```python
from build123d import *

# Parameters (mm, degrees)
EXTRUDE_1_DEPTH = 0.5
EXTRUDE_2_DEPTH = 0.2


with BuildPart() as part:
    # Эскиз1 → Бобышка-Вытянуть1 (new body)
    with BuildSketch(Plane.XY):
        with BuildLine():
            Line((25.396850198, 14), (-25.396850198, 14))
            ThreePointArc((-25.396850198, 14), (-29, 0), (-25.396850198, -14))
            Line((-25.396850198, -14), (25.396850198, -14))
            ThreePointArc((25.396850198, -14), (29, 0), (25.396850198, 14))
        make_face()
    extrude(amount=EXTRUDE_1_DEPTH)

    # Эскиз2 → Бобышка-Вытянуть2 (add)
    with BuildSketch(Plane(origin=(0, 0, 0), x_dir=(-1, 0, 0), z_dir=(0, 0, -1))):
        with BuildLine():
            Line((-24.494897428, -12.5), (24.494897428, -12.5))
            ThreePointArc((24.494897428, -12.5), (27.5, 0), (24.494897428, 12.5))
            Line((24.494897428, 12.5), (-24.494897428, 12.5))
            ThreePointArc((-24.494897428, 12.5), (-27.5, 0), (-24.494897428, -12.5))
        make_face()
    extrude(amount=EXTRUDE_2_DEPTH)


solid = part.part
```
The listing builds one solid part. Answer for the finished solid, in the listing's coordinates (mm). A direction names the side the tool comes from. Round coordinates to 2 decimals unless told otherwise and drop trailing zeros. Write each loop counter-clockwise with the first axis right and the second up, starting at its lowest first coordinate (ties: lowest second). Pieces come first, ordered by that corner, then holes. Notation, with made-up numbers: (-18, -24) -> (8, -24) arc R20 ccw to (8, -14) -> close; hole circle Ø8 at (67.25, -27). An arc over 180 degrees is marked (long way). Answer as a JSON object with one key per item and string values. Group by question number.
Q1. Section A-A (x = 11) is taken. Write down the section's boundary in (y, z), plus the area to 3 significant figures.
Q2. Which of the six approach directions +Z, -Z, +X, -X, +Y, -Y give full straight-line access (tool end or side, diameter ignored) to faces 1 (the face through (0, 0, -0.2)), 2 (the face through (-2, 13, 0))?
Q3. Section B-B (y = -5) is taken. Write down the section's boundary in (x, z), plus the area to 3 significant figures.
Q4. Section C-C (z = 0.35) is taken. Write down the section's boundary in (x, y).
Q5. Straight lines are drawn through the part: line 1 along X through (y, z) = (0.75, -0.15); line 2 along X through (y, z) = (12.75, 0.05). For each, find the intervals that lie inside material, in ascending order.
Check values:
{
 "1": {"outline": "(-14, 0) -> (-12.5, 0) -> (-12.5, -0.2) -> (12.5, -0.2) -> (12.5, 0) -> (14, 0) -> (14, 0.5) -> (-14, 0.5) -> close", "area": "19.0 mm^2"},
 "2": {"face 1": "-Z, +X, -X, +Y, -Y", "face 2": "-Z"},
 "3": {"outline": "(-28.57, 0) -> (-27.04, 0) -> (-27.04, -0.2) -> (27.04, -0.2) -> (27.04, 0) -> (28.57, 0) -> (28.57, 0.5) -> (-28.57, 0.5) -> close", "area": "39.4 mm^2"},
 "4": {"outline": "(-25.4, -14) -> (25.4, -14) arc R29 ccw to (25.4, 14) -> (-25.4, 14) arc R29 ccw to start"},
 "5": {"line 1": "-27.49 to 27.49", "line 2": "-26.05 to 26.05"}
}
